Geometry check sheet. Reference: the model listing, model coordinates, mm. A direction names the side the tool comes from. Give positions to 0.01 mm unless a question says otherwise; leave off trailing zeros. Loops run counter-clockwise (first coordinate to the right, second up) from the corner with the lowest first, then second, coordinate; pieces in that order, holes last. Notation, with made-up numbers: (11.5, 67.25) - (18.5, 67.25) arc R19 cw to (18.5, 74.25) - close; hole circle Ø1 at (-36, 1.25). An arc over 180 degrees is marked (long way). Use a Markdown table: item, result. Add a question column.
1. Draft check along Z on faces 6 (the flat face through (-17, -43, -15)), 7 (the cylindrical face through (-17.784, -30.432, -8.216)), 8 (the flat face through (-30, -37, 0)), 9 (the flat face through (-58, -76, -12)). Enter one of: pulls with the +Z half, pulls with the -Z half, needs draft (parallel to the pull), parting line crosses it, or undercut.
2. Cross-section at D-D on y = -110. Enter the section's corners in (x, z).
3. Depth check by flat-ended pin: P1, Ø5, axis at x = -17, z = -6.5, coming from the -Y side; P2, Ø4, axis at x = -86.5, z = -23.5, coming from the +Y side; P3, Ø4, axis at x = -39.5, y = -53.5, coming from the -Z side. Enter the tip coordinate at first touch or a pass-through.
4. Material ranges on L1, parallel to Z at x = -86.5, y = -74.75; L2, parallel to Y at x = -34, z = -4; L3, parallel to X at y = -74.55, z = -36, recorded low to high.
5. Cross-section at A-A on z = -31. Enter the section's corners in (x, y).
6. Cross-section at C-C on y = -36.5. Enter the section's corners in (x, z), and give its area (3 significant figures).
7. Set-up check for faces 1 (the flat face through (-59, -73, -12)), 2 (the flat face through (-57, 3, -12)), 3 (the cylindrical face through (-13.48, -15.46, -6.31)), 4 (the flat face through (24.65, 23.08, -7.4)), 5 (the cylindrical face through (-31.94, -11.96, -1.01)): record each of +Z, -Z, +X, -X, +Y, -Y from which the full face is reachable in a straight line by a thin tool's end or side.
8. Cross-section at B-B on x = -62.5. Enter the section's corners in (y, z).
from build123d import *

# Parameters (mm, degrees)
SKETCH1_R            = 1.5
BOSS_EXTRUDE1_DEPTH  = 3
BOSS_EXTRUDE2_DEPTH  = 15
BOSS_EXTRUDE4_DEPTH  = 2
CUT_SWEEP1_START     = -39.833089264
CUT_SWEEP1_OUTLINE_R = 2
CUT_SWEEP1_DEPTH     = 5.418212301
SKETCH13_R           = 2
CUT_EXTRUDE1_REACH   = 160.497
SKETCH14_R           = 2.5
SKETCH15_R           = 2.5
BOSS_EXTRUDE5_DEPTH  = 10
SKETCH16_R           = 2.5
CUT_EXTRUDE2_DEPTH   = 10


# Read off the part's stored shape, not the designer's step: Cut-Sweep1
with BuildPart() as part:
    # Sketch1 → Boss-Extrude1 (new body)
    with BuildSketch(Plane(origin=(0, 0, 0), x_dir=(1, 0, 0), z_dir=(0, 1, 0))):
        Polygon((-90, 42), (-90, 0), (0, 0), (0, 15), (-75, 15), (-75, 42), align=None)
        with Locations(Location((-86.5, 36, 0), (0, 0, 270))):
            Circle(SKETCH1_R, mode=Mode.SUBTRACT)
        with Locations(Location((-86.5, 23.5, 0), (0, 0, 270))):
            Circle(SKETCH1_R, mode=Mode.SUBTRACT)
    extrude(amount=BOSS_EXTRUDE1_DEPTH)


with BuildPart() as body_2:
    # Mirror7: mirrored copy
    add(part.part.mirror(Plane.ZX.offset(-36.5)))


with BuildPart() as part_1:
    add(part.part)

    add(body_2.part)  # Boss-Extrude2 merges body 2
    # Sketch3 → Boss-Extrude2 (add)
    with BuildSketch(Plane.XY):
        with BuildLine():
            Line((0, 0), (50, 46.811448287))
            Line((50, 46.811448287), (47.26621142, 49.731448287))
            Line((47.26621142, 49.731448287), (-2.73378858, 2.92))
            ThreePointArc((-2.73378858, 2.92), (-20.424933424, -35.957501235), (-5.557687519, -76))
            Line((-5.557687519, -76), (45.907254912, -124.182969825))
            Line((45.907254912, -124.182969825), (50, -119.811448287))
            Line((50, -119.811448287), (0, -73))
            ThreePointArc((0, -73), (-15.82764275, -36.5), (0, 0))
        make_face()
    extrude(amount=-BOSS_EXTRUDE2_DEPTH)

    # Sketch4 → Boss-Extrude4 (add)
    with BuildSketch(Plane.XY):
        with BuildLine():
            Line((-8.143678765, -73), (-55.631592513, -73))
            Line((-55.631592513, -73), (-55.631592513, 0))
            Line((-55.631592513, 0), (-5.631592513, 0))
            ThreePointArc((-5.631592513, 0), (-20.427620409, -36.034060143), (-8.143678765, -73))
        make_face()
    extrude(amount=-BOSS_EXTRUDE4_DEPTH)

    # Cut-Sweep1 outline → Cut-Sweep1 (cut)
    with BuildSketch(Plane(origin=(0, 0, 0), x_dir=(-0.4226182617406999, 0.9063077870366498, 0), z_dir=(0.9063077870366498, 0.4226182617406999, 0)).offset(CUT_SWEEP1_START)):
        with Locations((-47.522096447, -8)):
            Circle(CUT_SWEEP1_OUTLINE_R)
    cut_sweep1 = extrude(amount=CUT_SWEEP1_DEPTH, mode=Mode.SUBTRACT)

    # Cut-Sweep2: sweep along a path in Sketch12
    with BuildLine(Plane(origin=(0, 0, -8), x_dir=(-1, 0, 0), z_dir=(0, 0, -1))) as cut_sweep2_path:
        Line((-34.17235725, -36.5), (20.427620409, -40.807723062))
    # Sketch13 → Cut-Sweep2 (sweep, cut)
    with BuildSketch(Plane(origin=(34.17235725, -36.5, -8), x_dir=(0, 0, 1), z_dir=(-0.9969021605356864, -0.07865165172633562, 0))):
        with Locations((0.218000658, -0.010354147)):
            Circle(SKETCH13_R)
    cut_sweep2 = sweep(path=cut_sweep2_path.line, mode=Mode.SUBTRACT)

    # Mirror8: Cut-Sweep1, Cut-Sweep2 across plane
    add(cut_sweep1.mirror(Plane.ZX.offset(-36.5)), mode=Mode.SUBTRACT)
    add(cut_sweep2.mirror(Plane.ZX.offset(-36.5)), mode=Mode.SUBTRACT)

    # Sketch14 → Cut-Extrude1 (cut, up to next)
    with BuildSketch(Plane(origin=(0, 0, -2), x_dir=(-1, 0, 0), z_dir=(0, 0, -1)), mode=Mode.PRIVATE) as cut_extrude1_sk1:
        with Locations((35.631592513, -36.5)):
            Circle(SKETCH14_R)
    cut_extrude1_tool1 = extrude(cut_extrude1_sk1.sketch, amount=-CUT_EXTRUDE1_REACH, mode=Mode.PRIVATE) & part_1.part
    add(cut_extrude1_tool1.solids().sort_by_distance((-35.631593, -36.5, -2))[0], mode=Mode.SUBTRACT)

    # Sketch15 → Boss-Extrude5 (add)
    with BuildSketch(Plane(origin=(0, 0, -2), x_dir=(-1, 0, 0), z_dir=(0, 0, -1))):
        with Locations(Location((40.631592513, -53, 0), (0, 0, 180))):
            Circle(SKETCH15_R)
    boss_extrude5 = extrude(amount=BOSS_EXTRUDE5_DEPTH)

    # Mirror9: Boss-Extrude5 across plane
    add(boss_extrude5.mirror(Plane.ZX.offset(-36.5)))

    # Sketch16 → Cut-Extrude2 (cut)
    with BuildSketch(Plane(origin=(0, 0, -2), x_dir=(-1, 0, 0), z_dir=(0, 0, -1))):
        with Locations((29.631592513, -11)):
            Circle(SKETCH16_R)
    cut_extrude2 = extrude(amount=-CUT_EXTRUDE2_DEPTH, mode=Mode.SUBTRACT)

    # Mirror10: Cut-Extrude2 across plane
    add(cut_extrude2.mirror(Plane.ZX.offset(-36.5)), mode=Mode.SUBTRACT)


solid = part_1.part
Values found:
| question | item | result |
|---|---|---|
| 1 | face 6 | pulls with the -Z half |
| 1 | face 7 | undercut |
| 1 | face 8 | pulls with the +Z half |
| 1 | face 9 | needs draft |
| 2 | outline | (30.76, -15) - (39.52, -15) - (39.52, 0) - (30.76, 0) - close |
| 3 | P1 | stops at y = -76 |
| 3 | P2 | stops at y = 3 |
| 3 | P3 | stops at z = -12 |
| 4 | L1 | z = -42 to -37.5, -34.5 to -25, -22 to 0 |
| 4 | L2 | y = -76 to -73, 0 to 3 |
| 4 | L3 | x = -90 to -88, -85 to -75 |
| 5 | outline | (-90, -76) - (-75, -76) - (-75, -73) - (-90, -73) - close; (-90, 0) - (-75, 0) - (-75, 3) - (-90, 3) - close |
| 6 | outline | (-55.63, -2) - (-38.13, -2) - (-38.13, 0) - (-55.63, 0) - close; (-33.13, -2) - (-20.44, -2) - (-20.44, -15) - (-15.83, -15) - (-15.83, 0) - (-33.13, 0) - close |
| 6 | area | 130 mm2 |
| 7 | face 1 | -Z, -X |
| 7 | face 2 | +Z, -Z, -X, +Y |
| 7 | face 3 | none |
| 7 | face 4 | +Z, -Z, +X |
| 7 | face 5 | +Z, -Z |
| 8 | outline | (-76, -15) - (-73, -15) - (-73, 0) - (-76, 0) - close; (0, -15) - (3, -15) - (3, 0) - (0, 0) - close |
